```python
from build123d import *

# Parameters (mm, degrees)
SKETCH_1_R          = 1.45
EXTRUDE_1_DEPTH     = 3
EXTRUDE_2_DEPTH     = 3
SKETCH_4_W          = 43.75
SKETCH_4_H          = 58.75
CUT_EXTRUDE_2_DEPTH = 79.02002948
FILLET_1_R          = 3


with BuildPart() as part:
    # 草图1 → 凸台-拉伸1 (new body)
    with BuildSketch(Plane(origin=(0, 0, 0), x_dir=(1, 0, 0), z_dir=(0, 1, 0))):
        Polygon((-51.25, 0), (0, 0), (51.25, 0), (51.25, -15), (7.5, -15), (7.5, -58.75), (-7.5, -58.75), (-7.5, -15), (-51.25, -15), align=None)
        with Locations(Location((0, -7.5, 0), (0, 0, 270))):
            Circle(SKETCH_1_R, mode=Mode.SUBTRACT)
        with Locations(Location((0, -33.75, 0), (0, 0, 270))):
            Circle(SKETCH_1_R, mode=Mode.SUBTRACT)
        with Locations(Location((0, -53.75, 0), (0, 0, 270))):
            Circle(SKETCH_1_R, mode=Mode.SUBTRACT)
        with Locations(Location((-26.25, -7.5, 0), (0, 0, 270))):
            Circle(SKETCH_1_R, mode=Mode.SUBTRACT)
        with Locations(Location((-46.25, -7.5, 0), (0, 0, 270))):
            Circle(SKETCH_1_R, mode=Mode.SUBTRACT)
        with Locations(Location((46.25, -7.5, 0), (0, 0, 90))):
            Circle(SKETCH_1_R, mode=Mode.SUBTRACT)
        with Locations(Location((26.25, -7.5, 0), (0, 0, 90))):
            Circle(SKETCH_1_R, mode=Mode.SUBTRACT)
    extrude(amount=EXTRUDE_1_DEPTH)

    # 草图2 → 凸台-拉伸2 (add)
    with BuildSketch(Plane(origin=(0, 3, 0), x_dir=(1, 0, 0), z_dir=(0, 1, 0))):
        Polygon((-51.25, -15), (-7.5, -58.75), (-7.5, -48.850505063), (-41.350505063, -15), align=None)
        Polygon((41.350505063, -15), (51.25, -15), (7.5, -58.75), (7.5, -48.850505063), align=None)
    extrude(amount=-EXTRUDE_2_DEPTH)

    # 草图4 → 切除-拉伸2 (cut, through all)
    with BuildSketch(Plane(origin=(0, 3, 0), x_dir=(1, 0, 0), z_dir=(0, 1, 0))):
        with Locations((29.375, -29.375)):
            Rectangle(SKETCH_4_W, SKETCH_4_H)
    extrude(amount=-CUT_EXTRUDE_2_DEPTH, mode=Mode.SUBTRACT)

    # 圆角1
    fillet_1_edges = [part.edges().sort_by_distance(p)[0] for p in [
        (-51.25, 1.5, 0),
        (7.5, 1.5, 58.75),
        (-7.5, 1.5, 58.75),
        (-7.5, 1.5, 15),
        (-51.25, 1.5, 15),
        (-7.5, 1.5, 48.850505063),
        (-41.350505063, 1.5, 15),
        (7.5, 1.5, 0),
    ]]
    fillet(fillet_1_edges, radius=FILLET_1_R)


solid = part.part
```
Work out the finished part from the listing and answer in its coordinate system (mm). A direction names the side the tool comes from. Give positions to 0.01 mm unless a question says otherwise; leave off trailing zeros. Loops run counter-clockwise (first coordinate to the right, second up) from the corner with the lowest first, then second, coordinate; pieces in that order, holes last. Notation, with made-up numbers: (2.25, -37) -> (25.25, -37) arc R11 cw to (25.25, -23) -> close; hole circle Ø5 at (62.25, -26.5). An arc over 180 degrees is marked (long way). Put each result on its own line as item: value. Start each with the question number.
Item 1: The mould has two halves that part along Z. Classify faces 1 (the face through (-8.36, 1.52, 15.9)), 2 (the face through (-22, 1, 0)), 3 (the face through (-22, 0, 35)): released by +Z, released by -Z, zero draft, split by the parting line, or undercut.
Item 2: The part is cut by section D-D (z = 53.75). Give the vertices of the cut face in (x, y).
Item 3: The part is cut by section A-A (x = 0). Give the vertices of the cut face in (y, z), then the cut area to 3 significant figures.
Item 4: Find the intervals of material crossed by L1, parallel to X at y = 1.45, z = 7.5; L2, parallel to Z at x = -1, y = 1.2; L3, parallel to X at y = 2.35, z = 33.75, in increasing order. Write a range as [from, to].
Item 5: The part is cut by section B-B (x = -46.25). Give the vertices of the cut face in (y, z), then the cut area to 3 significant figures.
Item 6: The part is cut by section C-C (y = 1.65). Give the vertices of the cut face in (x, z).
Item 7: Which of the six approach directions +Z, -Z, +X, -X, +Y, -Y give full straight-line access (tool end or side, diameter ignored) to faces 4 (the face through (-9.31, 1.48, 44.36)), 5 (the face through (6.6, 1.48, 0.86))?
Answers below:
1. face 1: undercut
1. face 2: released by -Z
1. face 3: zero draft
2. outline: (-12.5, 0) -> (-1.45, 0) -> (-1.45, 3) -> (-12.5, 3) -> close; (1.45, 0) -> (7.5, 0) -> (7.5, 3) -> (1.45, 3) -> close
3. outline: (0, 0) -> (3, 0) -> (3, 6.05) -> (0, 6.05) -> close; (0, 8.95) -> (3, 8.95) -> (3, 32.3) -> (0, 32.3) -> close; (0, 35.2) -> (3, 35.2) -> (3, 52.3) -> (0, 52.3) -> close; (0, 55.2) -> (3, 55.2) -> (3, 58.75) -> (0, 58.75) -> close
3. area: 150 mm2
4. L1: [-51.25, -47.7], [-44.8, -27.7], [-24.8, -1.45], [1.45, 7.5]
4. L2: [0, 6.45], [8.55, 32.7], [34.8, 52.7], [54.8, 58.75]
4. L3: [-32.5, -22.6], [-7.5, -1.45], [1.45, 7.5]
5. outline: (0, 0) -> (3, 0) -> (3, 6.05) -> (0, 6.05) -> close; (0, 8.95) -> (3, 8.95) -> (3, 20) -> (0, 20) -> close
5. area: 51.3 mm2
6. outline: (-51.25, 3) arc R3 ccw to (-48.25, 0) -> (4.5, 0) arc R3 ccw to (7.5, 3) -> (7.5, 55.75) arc R3 ccw to (4.5, 58.75) -> (-6.26, 58.75) arc R3 ccw to (-8.38, 57.87) -> (-50.37, 15.88) arc R3 ccw to (-51.25, 13.76) -> close; hole circle Ø2.9 at (-46.25, 7.5); hole (-36.23, 20.12) arc R3 ccw to (-34.11, 15) -> (-10.5, 15) arc R3 ccw to (-7.5, 18) -> (-7.5, 41.61) arc R3 ccw to (-12.62, 43.73) -> close; hole circle Ø2.9 at (-26.25, 7.5); hole circle Ø2.9 at (0, 7.5); hole circle Ø2.9 at (0, 33.75); hole circle Ø2.9 at (0, 53.75)
7. face 4: +Y, -Y
7. face 5: -Z, +X, +Y, -Y
